The listing builds one solid part. Answer for the finished solid, in the listing's coordinates (mm). Face numbers are marked on the shaded views. A direction names the side the tool comes from. Round coordinates to 2 decimals unless told otherwise and drop trailing zeros. Write each loop counter-clockwise with the first axis right and the second up, starting at its lowest first coordinate (ties: lowest second). Pieces come first, ordered by that corner, then holes.
(1) Each of these flat-tipped pins is pushed along its axis until it touches: pin 1 Ø3 at (x, z) = (8, 4) entering from +Y; pin 2 Ø8 at (y, z) = (-14.5, 7) entering from -X; pin 3 Ø2 at (x, z) = (-6, 8) entering from -Y. Where does it stop, or does it pass through?
(2) A cutting plane is placed at D-D, the plane y = 11. Give the vertices of the cut face in (x, z).
(3) The mould has two halves that part along Y. Classify the marked faces 3, 4 and 5: +Y half, -Y half, draft (parallel to the pull), parting line (faces both ways), or undercut.
(4) For the marked faces 1 and 2, determine the directions among +Z, -Z, +X, -X, +Y, -Y from which every point of the face is accessible in a straight line to the end or side of a thin tool.
(5) Find the intervals of material crossed by probe 1 along Y at (x, z) = (0, -0.75); probe 2 along Z at (x, y) = (16, 9.5); probe 3 along X at (y, z) = (-5, 2.25), in increasing order.
(6) A cutting plane is placed at C-C, the plane z = 2.75. Give the vertices of the cut face in (x, y).
(7) A cutting plane is placed at A-A, the plane y = 0. Give the vertices of the cut face in (x, z), and give its area (3 significant figures).
(8) A cutting plane is placed at B-B, the plane x = 0. Give the vertices of the cut face in (y, z), and give its area (3 significant figures).
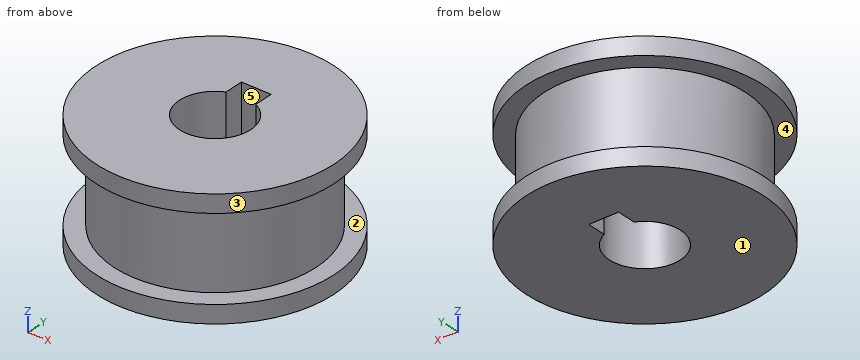
from build123d import *

# Parameters (mm, degrees)
SKETCH_1_R          = 17
EXTRUDE_1_DEPTH     = 10
SKETCH_2_R          = 20
EXTRUDE_2_DEPTH     = 3
CUT_EXTRUDE_1_DEPTH = 35.641016151


with BuildPart() as part:
    # 草图1 → 凸台-拉伸1 (new, symmetric)
    with BuildSketch(Plane.XY):
        Circle(SKETCH_1_R)
    extrude(amount=EXTRUDE_1_DEPTH, both=True)

    # 草图2 → 凸台-拉伸2 (add)
    with BuildSketch(Plane.XY.offset(10)):
        Circle(SKETCH_2_R)
    extrude_2 = extrude(amount=-EXTRUDE_2_DEPTH)

    # 镜向1: 凸台-拉伸2 across plane
    add(extrude_2.mirror(Plane.XY))

    # 草图3 → 切除-拉伸1 (cut, through all)
    with BuildSketch(Plane.XY.offset(10)):
        with BuildLine():
            Line((2.5, 8.68), (-2.5, 8.68))
            Line((-2.5, 8.68), (-2.5, 5.454356057))
            ThreePointArc((-2.5, 5.454356057), (0, -6), (2.5, 5.454356057))
            Line((2.5, 5.454356057), (2.5, 8.68))
        make_face()
    extrude(amount=-CUT_EXTRUDE_1_DEPTH, mode=Mode.SUBTRACT)


solid = part.part
Solutions:
1. pin 1: stops at y = 15.71
1. pin 2: stops at x = -17.02
1. pin 3: stops at y = -19.36
2. outline: (-16.7, -10) - (16.7, -10) - (16.7, -7) - (12.96, -7) - (12.96, 7) - (16.7, 7) - (16.7, 10) - (-16.7, 10) - (-16.7, 7) - (-12.96, 7) - (-12.96, -7) - (-16.7, -7) - close
3. face 3: parting line
3. face 4: draft
3. face 5: undercut
4. face 1: -Z, +X, -X, +Y, -Y
4. face 2: none
5. probe 1: y = -17 to -6, 8.68 to 17
5. probe 2: z = -10 to -7, 7 to 10
5. probe 3: x = -16.25 to -3.32, 3.32 to 16.25
6. outline: circle Ø34 at (0, 0); hole (-2.5, 5.45) arc R6 ccw (long way) to (2.5, 5.45) - (2.5, 8.68) - (-2.5, 8.68) - close
7. outline: (-20, -10) - (-6, -10) - (-6, 10) - (-20, 10) - (-20, 7) - (-17, 7) - (-17, -7) - (-20, -7) - close; (6, -10) - (20, -10) - (20, -7) - (17, -7) - (17, 7) - (20, 7) - (20, 10) - (6, 10) - close
7. area: 476 mm2
8. outline: (-20, -10) - (-6, -10) - (-6, 10) - (-20, 10) - (-20, 7) - (-17, 7) - (-17, -7) - (-20, -7) - close; (8.68, -10) - (20, -10) - (20, -7) - (17, -7) - (17, 7) - (20, 7) - (20, 10) - (8.68, 10) - close
8. area: 422 mm2
